Verification items for the finished model (mm, model axes). Give positions to 0.01 mm unless a question says otherwise; leave off trailing zeros. Order: outer loops, then holes, each group sorted by start corner. A loop starts at its lowest first (then second) coordinate and runs counter-clockwise, first axis right, second up.
(1) Sectioned sample at B-B on z = 0. Record the cut outline in (x, y), plus the area to 3 significant figures.
(2) Sectioned sample at D-D on x = -13. Record the cut outline in (y, z).
(3) Scan lines: L1, parallel to Z at x = 16.25, y = 1.15; L2, parallel to X at y = 1.95, z = 4.5; L3, parallel to Z at x = -23.5, y = 2.85. Record each from-to range of solid material in increasing order.
(4) Mould release check, pull along X, two halves, no side actions. Record for faces 1 (the face through (-31.58, 1.48, -23.89)), 2 (the face through (31.39, 1.48, -24.08)), 3 (the face through (22.744, 1.479, -0.286)): pulls with the +X half, pulls with the -X half, needs draft (parallel to the pull), parting line crosses it, or undercut.
(5) Sectioned sample at C-C on y = 1.45. Record the cut outline in (x, z), plus the area to 3 significant figures.
(6) Sectioned sample at A-A on x = 16.25. Record the cut outline in (y, z), plus the area to 3 significant figures.
```python
from build123d import *

# Parameters (mm, degrees)
SKETCH1_W               = 70
SKETCH1_H               = 67
BOSS_EXTRUDE1_DEPTH     = 3
SKETCH5_W               = 70
SKETCH5_H               = 6
CUT_EXTRUDE4_DEPTH      = 1
CUT_EXTRUDE4_DEPTH_BACK = 4
FILLET1_R               = 12
CUT_EXTRUDE1_START      = -4
SKETCH2_R               = 6.5
CUT_EXTRUDE1_DEPTH      = 5


with BuildPart() as part:
    # Sketch1 → Boss-Extrude1 (new body)
    with BuildSketch(Plane(origin=(0, 0, 0), x_dir=(1, 0, 0), z_dir=(0, 1, 0))):
        Rectangle(SKETCH1_W, SKETCH1_H)
    extrude(amount=BOSS_EXTRUDE1_DEPTH)

    # Sketch5 → Cut-Extrude4 (cut, two sides)
    with BuildSketch(Plane(origin=(0, 3, 0), x_dir=(1, 0, 0), z_dir=(0, 1, 0))) as cut_extrude4_sk:
        with Locations((0, 30.5)):
            Rectangle(SKETCH5_W, SKETCH5_H)
    extrude(amount=CUT_EXTRUDE4_DEPTH, mode=Mode.SUBTRACT)
    extrude(cut_extrude4_sk.sketch, amount=-CUT_EXTRUDE4_DEPTH_BACK, mode=Mode.SUBTRACT)

    # Fillet1
    fillet1_edges = [part.edges().sort_by_distance(p)[0] for p in [
        (-35, 1.5, -27.5),
        (35, 1.5, -27.5),
    ]]
    fillet(fillet1_edges, radius=FILLET1_R)

    # Sketch2 → Cut-Extrude1 (cut)
    with BuildSketch(Plane(origin=(0, 3, 0), x_dir=(1, 0, 0), z_dir=(0, 1, 0)).offset(CUT_EXTRUDE1_START)):
        with Locations((-16.25, 0)):
            Circle(SKETCH2_R)
    cut_extrude1 = extrude(amount=CUT_EXTRUDE1_DEPTH, mode=Mode.SUBTRACT)

    # Mirror1: Cut-Extrude1 across plane
    add(cut_extrude1.mirror(Plane(origin=(0, 0, 0), x_dir=(0, 0, 1), z_dir=(1, 0, 0))), mode=Mode.SUBTRACT)


solid = part.part
```
Ans:
1. outline: (-35, 0) - (-22.75, 0) - (-22.75, 3) - (-35, 3) - close; (-9.75, 0) - (9.75, 0) - (9.75, 3) - (-9.75, 3) - close; (22.75, 0) - (35, 0) - (35, 3) - (22.75, 3) - close
1. area: 132 mm2
2. outline: (0, -27.5) - (3, -27.5) - (3, -5.63) - (0, -5.63) - close; (0, 5.63) - (3, 5.63) - (3, 33.5) - (0, 33.5) - close
3. L1: z = -27.5 to -6.5, 6.5 to 33.5
3. L2: x = -35 to -20.94, -11.56 to 11.56, 20.94 to 35
3. L3: z = -27.49 to 33.5
4. face 1: pulls with the -X half
4. face 2: pulls with the +X half
4. face 3: undercut
5. outline: (-35, -15.5) arc R12 ccw to (-23, -27.5) - (23, -27.5) arc R12 ccw to (35, -15.5) - (35, 33.5) - (-35, 33.5) - close; hole circle Ø13 at (-16.25, 0); hole circle Ø13 at (16.25, 0)
5. area: 3,940 mm2
6. outline: (0, -27.5) - (3, -27.5) - (3, -6.5) - (0, -6.5) - close; (0, 6.5) - (3, 6.5) - (3, 33.5) - (0, 33.5) - close
6. area: 144 mm2
